Input: part model. Units: mm. Frame: model coordinates. A direction names the side the tool comes from. Give positions to 0.01 mm unless a question says otherwise; leave off trailing zeros. Order: outer loops, then holes, each group sorted by start corner. A loop starts at its lowest first (then second) coordinate and runs counter-clockwise, first axis right, second up. Notation, with made-up numbers: M 52.25,77 L 57.25,77 A17 cw 57.25,82 Z; hole C 88.5,56.25 d11. An arc over 180 degrees is marked long. Use a Markdown table: item, result.
from build123d import *

# Parameters (mm, degrees)
SKETCH1_W           = 85
SKETCH1_H           = 58
BOSS_EXTRUDE1_DEPTH = 33
SKETCH2_W           = 11
SKETCH2_H           = 57
CUT_EXTRUDE1_DEPTH  = 32
SKETCH3_W           = 6
SKETCH3_H           = 57
CUT_EXTRUDE2_DEPTH  = 32
SKETCH4_W           = 9
SKETCH4_H           = 33
BOSS_EXTRUDE2_DEPTH = 20
CUT_EXTRUDE3_REACH  = 63.125
FILLET1_R           = 2


with BuildPart() as part:
    # Sketch1 → Boss-Extrude1 (new body)
    with BuildSketch(Plane(origin=(0, 0, 0), x_dir=(1, 0, 0), z_dir=(0, 1, 0))):
        Rectangle(SKETCH1_W, SKETCH1_H)
    extrude(amount=BOSS_EXTRUDE1_DEPTH)

    # Sketch2 → Cut-Extrude1 (cut)
    with BuildSketch(Plane(origin=(0, 33, 0), x_dir=(1, 0, 0), z_dir=(0, 1, 0))):
        with Locations((37, -0.5)):
            Rectangle(SKETCH2_W, SKETCH2_H)
    extrude(amount=-CUT_EXTRUDE1_DEPTH, mode=Mode.SUBTRACT)

    # Sketch3 → Cut-Extrude2 (cut)
    with BuildSketch(Plane(origin=(0, 33, 0), x_dir=(1, 0, 0), z_dir=(0, 1, 0))):
        with Locations((-39.5, -0.5)):
            Rectangle(SKETCH3_W, SKETCH3_H)
    extrude(amount=-CUT_EXTRUDE2_DEPTH, mode=Mode.SUBTRACT)

    # Sketch4 → Boss-Extrude2 (add)
    with BuildSketch(Plane(origin=(0, 1, 0), x_dir=(1, 0, 0), z_dir=(0, 1, 0))):
        with Locations((36, -2.5)):
            Rectangle(SKETCH4_W, SKETCH4_H)
    extrude(amount=BOSS_EXTRUDE2_DEPTH)

    # Sketch5 → Cut-Extrude3 (cut, up to next)
    with BuildSketch(Plane.XZ, mode=Mode.PRIVATE) as cut_extrude3_sk1:
        with BuildLine():
            Line((38.5, -25.5), (38.5, -23.5))
            Line((38.5, -23.5), (40.5, -23.5))
            ThreePointArc((40.5, -23.5), (37.085786438, -22.085786438), (38.5, -25.5))
        make_face()
    cut_extrude3_tool1 = extrude(cut_extrude3_sk1.sketch, amount=-CUT_EXTRUDE3_REACH, mode=Mode.PRIVATE) & part.part
    # Sketch5 → Cut-Extrude3 (cut, up to next)
    with BuildSketch(Plane.XZ, mode=Mode.PRIVATE) as cut_extrude3_sk2:
        with BuildLine():
            Line((40.5, -23.5), (38.5, -23.5))
            Line((38.5, -23.5), (38.5, -25.5))
            ThreePointArc((38.5, -25.5), (39.914213562, -24.914213562), (40.5, -23.5))
        make_face()
    cut_extrude3_tool2 = extrude(cut_extrude3_sk2.sketch, amount=-CUT_EXTRUDE3_REACH, mode=Mode.PRIVATE) & part.part
    # Sketch5 → Cut-Extrude3 (cut, up to next)
    with BuildSketch(Plane.XZ, mode=Mode.PRIVATE) as cut_extrude3_sk3:
        with BuildLine():
            Line((38.5, -25.5), (38.5, -23.5))
            Line((38.5, -23.5), (40.5, -23.5))
            ThreePointArc((40.5, -23.5), (37.085786438, -22.085786438), (38.5, -25.5))
        make_face()
    cut_extrude3_tool3 = extrude(cut_extrude3_sk3.sketch, amount=-CUT_EXTRUDE3_REACH, mode=Mode.PRIVATE) & part.part
    # Sketch5 → Cut-Extrude3 (cut, up to next)
    with BuildSketch(Plane.XZ, mode=Mode.PRIVATE) as cut_extrude3_sk4:
        with BuildLine():
            Line((40.5, -23.5), (38.5, -23.5))
            Line((38.5, -23.5), (38.5, -25.5))
            ThreePointArc((38.5, -25.5), (39.914213562, -24.914213562), (40.5, -23.5))
        make_face()
    cut_extrude3_tool4 = extrude(cut_extrude3_sk4.sketch, amount=-CUT_EXTRUDE3_REACH, mode=Mode.PRIVATE) & part.part
    # Sketch5 → Cut-Extrude3 (cut, up to next)
    with BuildSketch(Plane.XZ, mode=Mode.PRIVATE) as cut_extrude3_sk5:
        with BuildLine():
            Line((-39.5, 22), (-42.5, 22))
            ThreePointArc((-42.5, 22), (-44.5, 24), (-42.5, 26))
            Line((-42.5, 26), (-39.5, 26))
            ThreePointArc((-39.5, 26), (-37.5, 24), (-39.5, 22))
        make_face()
    cut_extrude3_tool5 = extrude(cut_extrude3_sk5.sketch, amount=-CUT_EXTRUDE3_REACH, mode=Mode.PRIVATE) & part.part
    add(cut_extrude3_tool1.solids().sort_by_distance((38.217058, 0, -23.217058))[0], mode=Mode.SUBTRACT)
    add(cut_extrude3_tool2.solids().sort_by_distance((39.348826, 0, -24.348826))[0], mode=Mode.SUBTRACT)
    add(cut_extrude3_tool3.solids().sort_by_distance((38.217058, 0, -23.217058))[0], mode=Mode.SUBTRACT)
    add(cut_extrude3_tool4.solids().sort_by_distance((39.348826, 0, -24.348826))[0], mode=Mode.SUBTRACT)
    add(cut_extrude3_tool5.solids().sort_by_distance((-41, 0, 24))[0], mode=Mode.SUBTRACT)

    # Fillet1
    fillet1_edges = [part.edges().sort_by_distance(p)[0] for p in [
        (-42.5, 33, -28.5),
        (42.5, 33, -28.5),
        (42.5, 0.5, 29),
        (31.5, 33, 0.5),
        (31.5, 17, 29),
        (-2.5, 33, 29),
        (-42.5, 0.5, 29),
        (-36.5, 17, 29),
    ]]
    fillet(fillet1_edges, radius=FILLET1_R)


solid = part.part
1) Reachability of faces 1 (the face through (36, 11, -14)), 2 (the face through (30.93, 32.4, -0.89)), 3 (the face through (-35.9, 16.78, 28.43)) from +Z, -Z, +X, -X, +Y, -Y: full face, straight path, thin tool, end or side. Return the list, or none.
Response values:
| item | result |
|---|---|
| face 1 | +X, +Y |
| face 2 | +Z, +X, +Y |
| face 3 | +Z, -X, +Y |
2) First-contact query: pin 1 Ø1 at (y, z) = (8, -2.5) entering from +X; pin 2 Ø7 at (x, z) = (34.5, 4.5) entering from +Y; pin 3 Ø10 at (x, y) = (35.5, 15) entering from +Z; pin 4 Ø2.5 at (x, z) = (38.5, -23.5) entering from +Y. Flat tips, straight axial feed; report the tip coordinate or a pass-through.
Response values:
| item | result |
|---|---|
| pin 1 | stops at x = 40.5 |
| pin 2 | stops at y = 32.32 |
| pin 3 | stops at z = 28.73 |
| pin 4 | passes through |
3) Cut plane D-D on y = 25. Return loops of the section in (x, z).
Response values:
| item | result |
|---|---|
| outline | M -42.5,-29 L 42.5,-29 L 42.5,-28 L 31.5,-28 L 31.5,27 A2 ccw 29.5,29 L -34.5,29 A2 ccw -36.5,27 L -36.5,-28 L -42.5,-28 Z |
4) Cut plane C-C on z = 24. Return loops of the section in (x, y), and give its area (3 significant figures).
Response values:
| item | result |
|---|---|
| outline | M -37.5,0 L 42.5,0 L 42.5,1 L 31.5,1 L 31.5,31 A2 ccw 29.5,33 L -36.5,33 L -36.5,1 L -37.5,1 Z |
| area | 2,260 mm² |
5) Cut plane A-A on z = 3.5. Return loops of the section in (x, y), and give its area (3 significant figures).
Response values:
| item | result |
|---|---|
| outline | M -42.5,0 L 42.5,0 L 42.5,1 L 40.5,1 L 40.5,21 L 31.5,21 L 31.5,31 A2 ccw 29.5,33 L -36.5,33 L -36.5,1 L -42.5,1 Z |
| area | 2,440 mm² |
6) Cut plane B-B on y = 19. Return loops of the section in (x, z), and give its area (3 significant figures).
Response values:
| item | result |
|---|---|
| outline | M -42.5,-29 L 42.5,-29 L 42.5,-28 L 31.5,-28 L 31.5,-14 L 40.5,-14 L 40.5,19 L 31.5,19 L 31.5,27 A2 ccw 29.5,29 L -34.5,29 A2 ccw -36.5,27 L -36.5,-28 L -42.5,-28 Z |
| area | 4,260 mm² |
7) Mould query, pull axis Z, two halves, no side actions, for faces 4 (the face through (41.9, 0.51, 28.43)), 5 (the face through (-37.5, 0.5, 24)), 6 (the face through (-1, 16, -29)), 7 (the face through (36, 17, -28)). Classes: released by +Z, released by -Z, zero draft, split by the parting line, or undercut.
Response values:
| item | result |
|---|---|
| face 4 | released by +Z |
| face 5 | undercut |
| face 6 | released by -Z |
| face 7 | undercut |
8) Material intervals for line 1 (Z direction, x = 32.5, y = 5); line 2 (X direction, y = 0.25, z = -23.5); line 3 (Z direction, x = 38.5, y = 0.7), sorted ascending. Write a range as from..to.
Response values:
| item | result |
|---|---|
| line 1 | z = -29..-28, -14..19 |
| line 2 | x = -42.5..36.5, 40.5..42.5 |
| line 3 | z = -29..-25.5, -21.5..29 |
